Work out the finished part from the listing and answer in its coordinate system (mm). A direction names the side the tool comes from. Round coordinates to 2 decimals unless told otherwise and drop trailing zeros. Write each loop counter-clockwise with the first axis right and the second up, starting at its lowest first coordinate (ties: lowest second). Pieces come first, ordered by that corner, then holes. Notation, with made-up numbers: (74.25, -1) -> (117.25, -1) arc R24 cw to (117.25, 35) -> close; hole circle Ø2 at (-3, 52). An arc over 180 degrees is marked (long way). Answer as a JSON object with one key per item and string values. Group by question number.
Autodesk Inventor part; units mm, degrees
ref_plane "YZ Plane" through (0, 0, 0) normal (1, 0, 0) x (0, 1, 0)
ref_plane "XZ Plane" through (0, 0, 0) normal (0, 1, 0) x (-1, 0, 0)
ref_plane "XY Plane" through (0, 0, 0) normal (0, 0, 1) x (1, 0, 0)
sketch "Sketch4" plane through (0, 0, 0) normal (0, 0, 1) x (1, 0, 0)
  circle A0 centre (0, 0) radius 3.1 construction
  line L0 (0, 0) -> (3.1, 0) construction
  line L1 (0, 0) -> (1.55, 2.6847) construction
  line L2 (0, 0) -> (-1.55, 2.6847) construction
  line L3 (0, 0) -> (-3.1, 0) construction
  line L4 (0, 0) -> (-1.55, -2.6847) construction
  line L5 (0, 0) -> (1.55, -2.6847) construction
  line L6 (-1.55, 2.6847) -> (1.55, 2.6847) construction
  line L7 (1.55, 2.6847) -> (3.1, 0) construction
  line L8 (3.1, 0) -> (1.55, -2.6847) construction
  line L9 (1.55, -2.6847) -> (-1.55, -2.6847) construction
  line L10 (-1.55, -2.6847) -> (-3.1, 0) construction
  line L11 (-3.1, 0) -> (-1.55, 2.6847) construction
  line L12 (3.6196, 0) -> (1.8098, 3.1347)
  line L13 (1.8098, 3.1347) -> (-1.8098, 3.1347)
  line L14 (-1.8098, 3.1347) -> (-3.6196, 0)
  line L15 (-3.6196, 0) -> (-1.8098, -3.1347)
  line L16 (-1.8098, -3.1347) -> (1.8098, -3.1347)
  line L17 (1.8098, -3.1347) -> (3.6196, 0)
  line L18 (2.6758, 4.6347) -> (5.3517, 0)
  line L19 (5.3517, 0) -> (2.6758, -4.6347)
  line L20 (2.6758, -4.6347) -> (-2.6758, -4.6347)
  line L21 (-2.6758, -4.6347) -> (-5.3517, 0)
  line L22 (-5.3517, 0) -> (-2.6758, 4.6347)
  line L23 (-2.6758, 4.6347) -> (2.6758, 4.6347)
  dimension "d8" = 6.2
  dimension "d11" = 360
  dimension "d13" = 0.45
  dimension "d14" = 1.5
extrude "Extrusion3" add sketch "Sketch4" along normal blind 8
sketch "Sketch5" plane through (-2.6758, 4.6347, 0) normal (0, 1, 0) x (1, 0, 0)
  line L0 (5.3517, 0) -> (0, 0)
  line L1 (0, 0) -> (0, -8)
  line L2 (5.3517, -8) -> (0, -8)
  line L3 (5.3517, 0) -> (5.3517, -8)
  circle A0 centre (2.6758, -5.5) radius 0.65
  circle A1 centre (2.6758, -2.5) radius 0.65
  line L4 (5.3517, -8) -> (0, -8)
  point P0 (2.6758, 0)
  point P1 (2.6758, -8)
  point P2 (2.6758, -8)
  dimension "d17" = 1.3
  dimension "d18" = 2.5
  dimension "d19" = 2.5
extrude "Extrusion4" cut sketch "Sketch5" against normal blind 10 contours A0 | A1
properties part number "hombro_nuevo"
1) For a pull along Z with two mould halves and no side action, classify faces 3 (the face through (2.727, 1.545, 3.944)), 4 (the face through (-0.085, -3.874, 4.856)), 5 (the face through (-0.141, -3.874, 3.135)), 6 (the face through (3.5, 1.1, 8)) as released by +Z, released by -Z, zero draft, split by the parting line, or undercut.
2) This flat-tipped pin is pushed along its axis until it touches: P1, Ø2, axis at y = 3.5, z = 5.5, coming from the -X side. Where does it stop, or does it pass through?
3) A cutting plane is placed at A-A on x = 0. Determine the outline of the cut face in (y, z).
4) A cutting plane is placed at C-C on x = 3. Determine the outline of the cut face in (y, z), plus the area to 3 significant figures.
5) A tool of negligible diameter and unlimited length cuts with its end or side. For faces 1 (the face through (0, -3.135, 4)), 2 (the face through (-3.995, -2.35, 3.944)), from which of +Z, -Z, +X, -X, +Y, -Y can it reach the whole face along a straight path? Write none if from no direction.
6) A cutting plane is placed at D-D on z = 5.75. Determine the outline of the cut face in (x, y).
7) A cutting plane is placed at B-B on z = 1.5. Determine the outline of the cut face in (x, y), plus the area to 3 significant figures.
8) Straight lines are drawn through the part: L1, parallel to Y at x = -1, z = 0.5; L2, parallel to Z at x = 0, y = 3.55; L3, parallel to X at y = -1, z = 7.5. For each, find the intervals that lie inside material, in ascending order.
Established:
{
 "1": {"face 3": "zero draft", "face 4": "undercut", "face 5": "undercut", "face 6": "released by +Z"},
 "2": {"P1": "stops at x = -3.91"},
 "3": {"outline": "(-4.63, 0) -> (-3.13, 0) -> (-3.13, 1.85) -> (-4.63, 1.85) -> close; (-4.63, 3.15) -> (-3.13, 3.15) -> (-3.13, 4.85) -> (-4.63, 4.85) -> close; (-4.63, 6.15) -> (-3.13, 6.15) -> (-3.13, 8) -> (-4.63, 8) -> close; (3.13, 0) -> (4.63, 0) -> (4.63, 1.85) -> (3.13, 1.85) -> close; (3.13, 3.15) -> (4.63, 3.15) -> (4.63, 4.85) -> (3.13, 4.85) -> close; (3.13, 6.15) -> (4.63, 6.15) -> (4.63, 8) -> (3.13, 8) -> close"},
 "4": {"outline": "(-4.07, 0) -> (-1.07, 0) -> (-1.07, 8) -> (-4.07, 8) -> close; (1.07, 0) -> (4.07, 0) -> (4.07, 8) -> (1.07, 8) -> close", "area": "48.0 mm²"},
 "5": {"face 1": "+Z, -Z", "face 2": "+Z, -Z, -X, -Y"},
 "6": {"outline": "(-5.35, 0) -> (-2.68, -4.63) -> (-0.6, -4.63) -> (-0.6, -3.13) -> (-1.81, -3.13) -> (-3.62, 0) -> (-1.81, 3.13) -> (-0.6, 3.13) -> (-0.6, 4.63) -> (-2.68, 4.63) -> close; (0.6, -4.63) -> (2.68, -4.63) -> (5.35, 0) -> (2.68, 4.63) -> (0.6, 4.63) -> (0.6, 3.13) -> (1.81, 3.13) -> (3.62, 0) -> (1.81, -3.13) -> (0.6, -3.13) -> close"},
 "7": {"outline": "(-5.35, 0) -> (-2.68, -4.63) -> (2.68, -4.63) -> (5.35, 0) -> (2.68, 4.63) -> (-2.68, 4.63) -> close; hole (-3.62, 0) -> (-1.81, -3.13) -> (1.81, -3.13) -> (3.62, 0) -> (1.81, 3.13) -> (-1.81, 3.13) -> close", "area": "40.4 mm²"},
 "8": {"L1": "y = -4.63 to -3.13, 3.13 to 4.63", "L2": "z = 0 to 1.85, 3.15 to 4.85, 6.15 to 8", "L3": "x = -4.77 to -3.04, 3.04 to 4.77"}
}
